Autodesk Inventor part; units mm, degrees
ref_plane "YZ Plane" through (0, 0, 0) normal (1, 0, 0) x (0, 1, 0)
ref_plane "XZ Plane" through (0, 0, 0) normal (0, 1, 0) x (-1, 0, 0)
ref_plane "XY Plane" through (0, 0, 0) normal (0, 0, 1) x (1, 0, 0)
sketch "Sketch1" plane through (0, 0, 0) normal (0, 0, 1) x (1, 0, 0)
  line L0 (0, 0) -> (13, 0)
  line L1 (13, 0) -> (13, 28.45)
  line L2 (13, 28.45) -> (0, 28.45)
  line L3 (0, 28.45) -> (0, 0)
  dimension "d0" = 13
  dimension "d1" = 28.45
extrude "Extrusion1" add sketch "Sketch1" along normal blind 26.7
sketch "Sketch2" plane through (0, 0, 26.7) normal (0, 0, 1) x (1, 0, 0)
  line L0 (13, 28.45) -> (0, 28.45)
  circle A0 centre (6.5, 19.07) radius 2.5
  point P0 (0, 0)
  dimension "d5" = 5
extrude "Extrusion2" add sketch "Sketch2" along normal blind 5
properties part number "servoRep"
Model file for the job. Use its own axes, mm. A direction names the side the tool comes from. Coordinates: 2 decimals unless noted, no trailing zeros. Loops run counter-clockwise (first coordinate to the right, second up) from the corner with the lowest first, then second, coordinate; pieces in that order, holes last. Notation, with made-up numbers: (52.5, 75.25) -> (83.5, 75.25) arc R9 cw to (83.5, 86.25) -> close; hole circle Ø2 at (-31.75, 52). An arc over 180 degrees is marked (long way). Use one line per item in the form item = value. Start each with the question number.
(1) Cut at D-D on y = 5.5. Give the cut face in (x, z), and give its area (3 significant figures).
(2) Cut at B-B on y = 17.75. Give the cut face in (x, z).
(3) Probe probe 1 along Z at (x, y) = (10.25, 11). List the from-to ranges inside material, lowest first. Write a range as from..to.
(4) Cut at C-C on z = 27.5. Give the cut face in (x, y), and give its area (3 significant figures).
(5) Pull direction Z, two halves, no side cores. Call faces 1 (the flat face through (6, 19, 31.7)), 2 (the flat face through (6, 14, 0)), 3 (the flat face through (0, 14, 13)): pulls with the +Z half, pulls with the -Z half, needs draft (parallel to the pull), parting line crosses it, or undercut.
(6) Flat gauge pins, fed straight in: pin 1 (5 mm diameter, centred on x = 2, y = 8.5, fed in from +Z); pin 2 (4 mm diameter, centred on x = 8, z = 9.5, fed in from -Y). Where does each tip first touch, or does it go through?
(7) Cut at A-A on x = 6.5. Give the cut face in (y, z), and give its area (3 significant figures).
(8) Tool access for faces 4 (the flat face through (13, 14, 13)), 5 (the cylindrical face through (5.96, 21.51, 29.16)): list every direction of +Z, -Z, +X, -X, +Y, -Y with a clear straight run to the whole face (end or side of a thin tool).
Values:
q1.outline = (0, 0) -> (13, 0) -> (13, 26.7) -> (0, 26.7) -> close
q1.area = 347 mm2
q2.outline = (0, 0) -> (13, 0) -> (13, 26.7) -> (8.62, 26.7) -> (8.62, 31.7) -> (4.38, 31.7) -> (4.38, 26.7) -> (0, 26.7) -> close
q3.probe_1 = 0..26.7
q4.outline = circle Ø5 at (6.5, 19.07)
q4.area = 19.6 mm2
q5.face_1 = pulls with the +Z half
q5.face_2 = pulls with the -Z half
q5.face_3 = needs draft
q6.pin_1 = 26.7
q6.pin_2 = 0
q7.outline = (0, 0) -> (28.45, 0) -> (28.45, 26.7) -> (21.57, 26.7) -> (21.57, 31.7) -> (16.57, 31.7) -> (16.57, 26.7) -> (0, 26.7) -> close
q7.area = 785 mm2
q8.face_4 = +Z, -Z, +X, +Y, -Y
q8.face_5 = +Z
